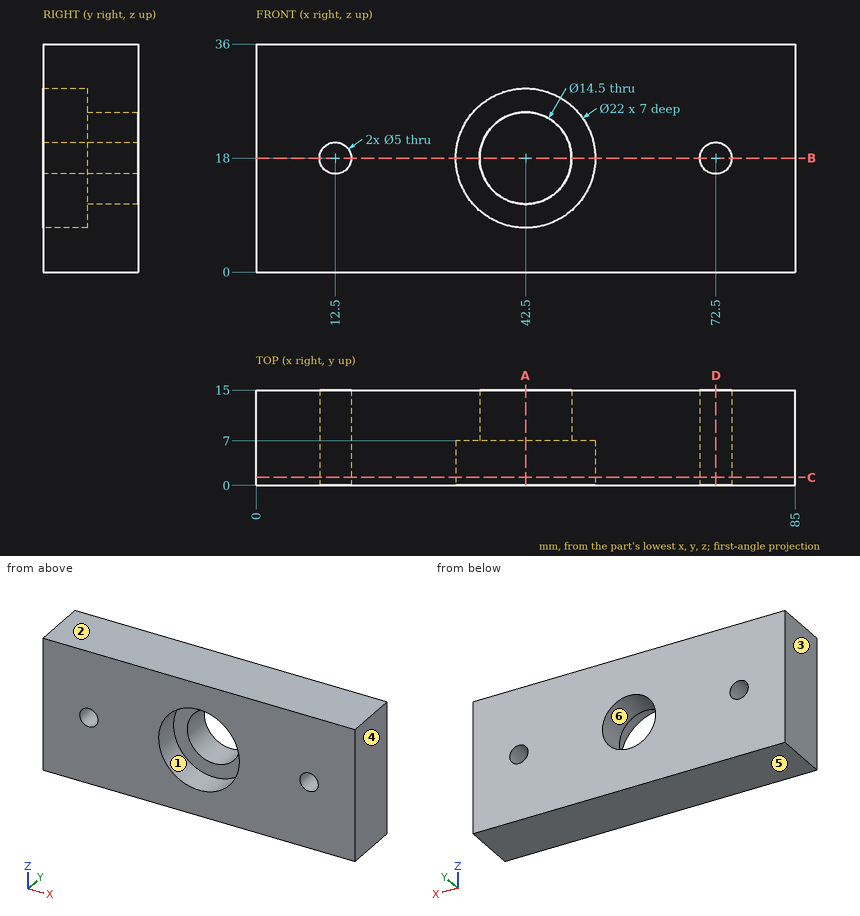
Input: dimensioned drawing with shaded views. Units: mm. Origin: part minimum x, y, z. A direction names the side the tool comes from. Round coordinates to 2 decimals unless told otherwise and drop trailing zeros. Order: outer loops, then holes, each group sorted by start corner. A loop starts at its lowest first (then second) coordinate and runs counter-clockwise, first axis right, second up. Notation, with made-up numbers: (53.5, 38) - (76.5, 38) arc R32 cw to (76.5, 64) - close; hole circle Ø3 at (61.5, 88). An arc over 180 degrees is marked (long way). Answer as a JSON object with one key per item and string values. Group by question number.
(1) Draft query along X for the marked faces 3, 4, 5 and 6. Return one class per face: released by +X, released by -X, zero draft, split by the parting line, or undercut.
(2) Material intervals for probe 1 along X at (y, z) = (3.5, 18); probe 2 along Z at (x, y) = (43, 9); probe 3 along X at (y, z) = (10.25, 17), sorted ascending. Write a range as from..to.
(3) Pin query (flat end, axial travel): P1, Ø2, axis at y = 12.5, z = 7.5, coming from the -X side; P2, Ø11, axis at x = 46.5, z = 15, coming from the -Y side. Return the tip coordinate at first contact, or that it passes through.
(4) Cut plane B-B (z = 18). Return loops of the section in (x, y), then the cut area to 3 significant figures.
(5) Cut plane A-A (x = 42.5). Return loops of the section in (y, z).
(6) Reachability of the marked faces 1 and 2 from +Z, -Z, +X, -X, +Y, -Y: full face, straight path, thin tool, end or side. Return the list, or none.
(7) Cut plane C-C (y = 1.25). Return loops of the section in (x, z), then the cut area to 3 significant figures.
(8) Cut plane D-D (x = 72.5). Return loops of the section in (y, z), then the cut area to 3 significant figures.
Here are the results:
{
 "1": {"face 3": "released by -X", "face 4": "released by +X", "face 5": "zero draft", "face 6": "undercut"},
 "2": {"probe 1": "x = 0..10, 15..31.5, 53.5..70, 75..85", "probe 2": "z = 0..10.77, 25.23..36", "probe 3": "x = 0..10.21, 14.79..35.32, 49.68..70.21, 74.79..85"},
 "3": {"P1": "stops at x = 0", "P2": "stops at y = 7"},
 "4": {"outline": "(0, 0) - (10, 0) - (10, 15) - (0, 15) - close; (15, 0) - (31.5, 0) - (31.5, 7) - (35.25, 7) - (35.25, 15) - (15, 15) - close; (49.75, 7) - (53.5, 7) - (53.5, 0) - (70, 0) - (70, 15) - (49.75, 15) - close; (75, 0) - (85, 0) - (85, 15) - (75, 15) - close", "area": "855 mm^2"},
 "5": {"outline": "(0, 0) - (15, 0) - (15, 10.75) - (7, 10.75) - (7, 7) - (0, 7) - close; (0, 29) - (7, 29) - (7, 25.25) - (15, 25.25) - (15, 36) - (0, 36) - close"},
 "6": {"face 1": "-Y", "face 2": "+Z, +X, -X, +Y, -Y"},
 "7": {"outline": "(0, 0) - (85, 0) - (85, 36) - (0, 36) - close; hole circle Ø5 at (12.5, 18); hole circle Ø22 at (42.5, 18); hole circle Ø5 at (72.5, 18)", "area": "2,640 mm^2"},
 "8": {"outline": "(0, 0) - (15, 0) - (15, 15.5) - (0, 15.5) - close; (0, 20.5) - (15, 20.5) - (15, 36) - (0, 36) - close", "area": "465 mm^2"}
}
